The listing builds one solid part. Answer for the finished solid, in the listing's coordinates (mm). Face numbers are marked on the shaded views. A direction names the side the tool comes from. Round coordinates to 2 decimals unless told otherwise and drop trailing zeros. Write each loop counter-clockwise with the first axis right and the second up, starting at its lowest first coordinate (ties: lowest second). Pieces come first, ordered by that corner, then holes. Notation, with made-up numbers: (-9, 31) - (47, 31) arc R36 ccw to (47, 67) - close; hole circle Ø8 at (43, 71.25). An arc over 180 degrees is marked (long way). Use a Markdown table: item, result. Add a question column.
1) A cutting plane is placed at B-B (z = 0). Give the vertices of the cut face in (x, y), then the cut area to 3 significant figures.
2) Determine the mould class of the marked faces 1, 2 and 3 for opening direction X: +X half, -X half, draft (parallel to the pull), parting line (faces both ways), or undercut.
3) A cutting plane is placed at C-C (y = 2.5). Give the vertices of the cut face in (x, z).
4) A cutting plane is placed at A-A (x = 0). Give the vertices of the cut face in (y, z).
5) Each of these flat-tipped pins is pushed along its axis until it touches: P1, Ø1.7, axis at x = -0.5, z = 0, coming from the +Y side; P2, Ø1.5, axis at x = 1, y = 0.5, coming from the -Z side. Where does it stop, or does it pass through?
6) A tool of negligible diameter and unlimited length cuts with its end or side. For the marked faces 4 and 5, from which of +Z, -Z, +X, -X, +Y, -Y can it reach the whole face along a straight path? Write none if from no direction.
7) Find the intervals of material crossed by probe 1 along Z at (x, y) = (0, 1.35); probe 2 along Z at (x, y) = (0, 0.3); probe 3 along X at (y, z) = (2.8, 1), in increasing order. Write a range as from..to.
Autodesk Inventor part; units mm, degrees
ref_plane "YZ Plane" through (0, 0, 0) normal (1, 0, 0) x (0, 1, 0)
ref_plane "XZ Plane" through (0, 0, 0) normal (0, 1, 0) x (-1, 0, 0)
ref_plane "XY Plane" through (0, 0, 0) normal (0, 0, 1) x (1, 0, 0)
sketch "Эскиз1" plane through (0, 0, 0) normal (0, 1, 0) x (-1, 0, 0)
  circle A0 centre (0, 0) radius 3.9
  circle A1 centre (0, 0) radius 2
  dimension "d0" = 7.8
  dimension "d1" = 4
extrude "Выдавливание1" add sketch "Эскиз1" along normal blind 3.1
sketch "Эскиз2" plane through (0, 3.1, 0) normal (0, 1, 0) x (1, 0, 0)
  circle A0 centre (0, 0) radius 3
  circle A1 centre (0, 0) radius 2.9
  circle A2 centre (0, 0) radius 3.9
  circle A3 centre (0, 0) radius 2
  dimension "d4" = 1
  dimension "d5" = 1
extrude "Выдавливание2" cut sketch "Эскиз2" against normal blind 0.5 contours A1 | A3
sketch "Эскиз3" plane through (0, 0, 0) normal (0, -1, 0) x (1, 0, 0)
  circle A0 centre (0, 0) radius 2.9
  circle A1 centre (0, 0) radius 3
  circle A2 centre (0, 0) radius 2.9
  circle A3 centre (0, 0) radius 3.9
  circle A4 centre (0, 0) radius 2
  dimension "d13" = 1
  dimension "d14" = 1
extrude "Выдавливание3" cut sketch "Эскиз3" against normal blind 0.5 contours A0 | A4
chamfer "Фаска1" distance 0.2 angle 45 4 edges at (-2.9, 0, 0) (3.9, 0, 0) (3.9, 3.1, 0) (-2.9, 3.1, 0)
properties part number "Подшипник 626Z" material "Титан"
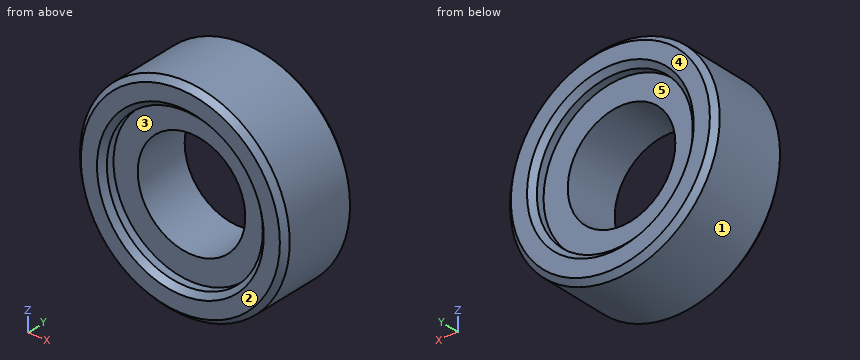
Entries:
| question | item | result |
|---|---|---|
| 1 | outline | (-3.9, 0.2) - (-3.7, 0) - (-3.1, 0) - (-2.9, 0.2) - (-2.9, 0.5) - (-2, 0.5) - (-2, 2.6) - (-2.9, 2.6) - (-2.9, 2.9) - (-3.1, 3.1) - (-3.7, 3.1) - (-3.9, 2.9) - close; (2, 0.5) - (2.9, 0.5) - (2.9, 0.2) - (3.1, 0) - (3.7, 0) - (3.9, 0.2) - (3.9, 2.9) - (3.7, 3.1) - (3.1, 3.1) - (2.9, 2.9) - (2.9, 2.6) - (2, 2.6) - close |
| 1 | area | 9.82 mm² |
| 2 | face 1 | parting line |
| 2 | face 2 | draft |
| 2 | face 3 | undercut |
| 3 | outline | circle Ø7.8 at (0, 0); hole circle Ø4 at (0, 0) |
| 4 | outline | (0, -3.7) - (0.2, -3.9) - (2.9, -3.9) - (3.1, -3.7) - (3.1, -3.1) - (2.9, -2.9) - (2.6, -2.9) - (2.6, -2) - (0.5, -2) - (0.5, -2.9) - (0.2, -2.9) - (0, -3.1) - close; (0, 3.1) - (0.2, 2.9) - (0.5, 2.9) - (0.5, 2) - (2.6, 2) - (2.6, 2.9) - (2.9, 2.9) - (3.1, 3.1) - (3.1, 3.7) - (2.9, 3.9) - (0.2, 3.9) - (0, 3.7) - close |
| 5 | P1 | passes through |
| 5 | P2 | stops at z = -3.89 |
| 6 | face 4 | +Z, -Z, +X, -X, +Y |
| 6 | face 5 | +Y |
| 7 | probe 1 | z = -3.9..-2, 2..3.9 |
| 7 | probe 2 | z = -3.9..-2.9, 2.9..3.9 |
| 7 | probe 3 | x = -3.77..-2.72, 2.72..3.77 |
